Solid Edge part; units mm, degrees
sketch "Sketch1" plane through (0, 0, 0) normal (0, -1, 0) x (1, 0, 0)
  line L0 (75, 75) -> (75, 0)
  line L1 (0, 0) -> (75, 0)
  arc A0 (75, 75) -> (0, 0) centre (75, 0) ccw
revolve "RevolvedProtrusion1" add sketch "Sketch1" angle 360 about axis through (0, 0, 0) along (1, 0, 0)
fillet "Round1" radius 2 1 edges at (75, 0, -75)
sketch "Sketch2" plane through (75, 0, 0) normal (1, 0, 0) x (0, 1, 0)
  line L0 (0, 6) -> (-45, 6)
  line L1 (0, 6) -> (45, 6)
  arc A0 (45, 6) -> (45, -6) centre (45, 0) cw
  line L2 (-45, -6) -> (45, -6)
  arc A1 (-45, -6) -> (-45, 6) centre (-45, 0) cw
extrude "ExtrudedCutout_1" cut sketch "Sketch2" against normal blind 5.8387
sketch "Sketch3" plane through (0, 0, -75.2808) normal (0, 0, 1) x (1, 0, 0)
  circle A0 centre (54.9452, 0) radius 18
extrude "ExtrudedProtrusion_4" add sketch "Sketch3" along normal blind 29
sketch "Sketch4" plane through (0, 0, -75.2808) normal (0, 0, 1) x (1, 0, 0)
  circle A0 centre (54.9452, 0) radius 18
extrude "ExtrudedProtrusion_3" add sketch "Sketch4" against normal blind 55.2919
sketch "Sketch5" plane through (75, 0, 0) normal (1, 0, 0) x (0, 1, 0)
  line L0 (-45, 10) -> (45, 10)
  line L1 (45, -10) -> (-45, -10)
  arc A0 (45, 10) -> (45, -10) centre (45, 0) cw
  arc A1 (-45, -10) -> (-45, 10) centre (-45, 0) cw
extrude "ExtrudedCutout_3" cut sketch "Sketch5" against normal blind 6
Can you work these out from the model? Positions are in its coordinate system, mm. A direction names the side the tool comes from. Round coordinates to 2 decimals unless told otherwise and drop trailing zeros. Order: outer loops, then holes, each group sorted by start corner. A loop starts at its lowest first (then second) coordinate and runs counter-clockwise, first axis right, second up. Notation, with made-up numbers: M 19.25,83.5 L 41.25,83.5 A21 cw 41.25,87.5 Z; hole C 52,-40 d7. An arc over 180 degrees is marked long. Use a Markdown table: item, result.
1) Imagine slicing it at B-B (x = 11.5). List the corners of the cut face in (y, z) for me, then the cut area to 3 significant figures.
Geometry says:
| item | result |
|---|---|
| outline | C 0,0 d79.82 |
| area | 5,000 mm² |
2) On a 3-axis mill with a long thin cutter (end or side, diameter ignored), from which of +Z, -Z, +X, -X, +Y, -Y can I reach the whole of each face in a straight line? I mean faces 1 (the face through (75, -1, 15)), 2 (the face through (72, 55, 0)). Say none if no direction works.
Geometry says:
| item | result |
|---|---|
| face 1 | +Z, -Z, +X, +Y, -Y |
| face 2 | +X |
3) Imagine slicing it at A-A (z = -114). List the corners of the cut face in (x, y) for me.
Geometry says:
| item | result |
|---|---|
| outline | C 54.95,0 d36 |
4) Imagine slicing it at C-C (x = 53.5). List the corners of the cut face in (y, z) for me.
Geometry says:
| item | result |
|---|---|
| outline | M -17.94,-130.57 L 17.94,-130.57 L 17.94,-69.58 A71.85 ccw long -17.94,-69.58 Z |
5) I'm going to push flat-ended pins straight in: P1, Ø6, axis at x = 61, z = -65.5, coming from the +Y side; P2, Ø3, axis at x = 72, y = -13.5, coming from the +Z side; P3, Ø4, axis at x = 24.5, y = -33.5, coming from the -Z side. Where does each tip first touch, or does it pass through?
Geometry says:
| item | result |
|---|---|
| P1 | stops at y = 39.14 |
| P2 | stops at z = 73.98 |
| P3 | stops at z = -46.81 |
6) Imagine slicing it at D-D (x = 65.5). List the corners of the cut face in (y, z) for me, then the cut area to 3 significant figures.
Geometry says:
| item | result |
|---|---|
| outline | M -14.58,-130.57 L 14.58,-130.57 L 14.58,-72.95 A74.4 ccw long -14.58,-72.95 Z |
| area | 19,000 mm² |
7) If we mould it in two halves opening along Y, with no side actions, what happens to faces 3 (the face through (55, 0, -130.573)), 4 (the face through (36.963, -0.791, -98.062)), 5 (the face through (69, -1, 0))? For each: +Y half, -Y half, draft (parallel to the pull), parting line (faces both ways), or undercut.
Geometry says:
| item | result |
|---|---|
| face 3 | draft |
| face 4 | parting line |
| face 5 | undercut |
8) If I drill on line 1 along Z through (x, y) = (59, -2); line 2 along Y through (x, z) = (56, -88); line 3 along Y through (x, z) = (64.5, -101), over which ranges is the centre line in solid material (lowest first)?
Geometry says:
| item | result |
|---|---|
| line 1 | z = -130.57 to 73.25 |
| line 2 | y = -17.97 to 17.97 |
| line 3 | y = -15.25 to 15.25 |
